Work out the finished part from the listing and answer in its coordinate system (mm). Face numbers are marked on the shaded views. A direction names the side the tool comes from. Give positions to 0.01 mm unless a question says otherwise; leave off trailing zeros. Write each loop counter-clockwise with the first axis right and the second up, starting at its lowest first coordinate (ties: lowest second). Pieces come first, ordered by that corner, then holes. Notation, with made-up numbers: (19, 51) -> (23, 51) arc R10 ccw to (23, 70) -> close; hole circle Ø1 at (-7, -36). An arc over 180 degrees is marked (long way). Write item = value, one per line. Start each with the question number.
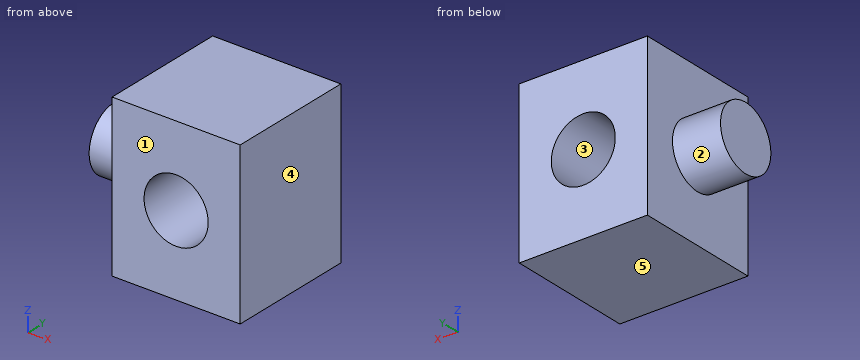
from build123d import *

# Parameters (mm, degrees)
F0_R     = 10
F1_DEPTH = 15
F0_W     = 40
F0_H     = 50
F2_DEPTH = 40
F3_R     = 10
F4_DEPTH = 40.001


with BuildPart() as f1:
    # F0 (on Right) → F1 (new body)
    with BuildSketch(Plane.YZ):
        Circle(F0_R)
    extrude(amount=-F1_DEPTH)

    # F0 (on Right) → F2 (join)
    with BuildSketch(Plane.YZ):
        Rectangle(F0_W, F0_H)
        Circle(F0_R, mode=Mode.SUBTRACT)
        Circle(F0_R)
    extrude(amount=F2_DEPTH)

    # F3 (on face) → F4 (cut, through all)
    with BuildSketch(Plane.XZ.offset(20)):
        with Locations((20, 0)):
            Circle(F3_R)
    extrude(amount=-F4_DEPTH, mode=Mode.SUBTRACT)


solid = f1.part
(1) Each of these flat-tipped pins is pushed along its axis until it touches: pin 1 (3 mm diameter, centred on x = -2.5, z = 16, fed in from -Y); pin 2 (1 mm diameter, centred on y = 15.5, z = 5.5, fed in from -X). Where does it stop, or does it pass through?
(2) Determine the mould class of the marked faces 3, 4 and 5 for opening direction Z: pulls with the +Z half, pulls with the -Z half, needs draft (parallel to the pull), parting line crosses it, or undercut.
(3) A cutting plane is placed at D-D, the plane y = -7.5. Write down the section's boundary in (x, z), then the cut area to 3 significant figures.
(4) Find the intervals of material crossed by line 1 along Z through (x, y) = (20, 2.5); line 2 along X through (y, z) = (-0.5, 13); line 3 along X through (y, z) = (8.5, -3.5), in increasing order.
(5) For the marked faces 1 and 2, determine the directions among +Z, -Z, +X, -X, +Y, -Y from which every point of the face is accessible in a straight line to the end or side of a thin tool.
(6) A cutting plane is placed at B-B, the plane x = 20. Write down the section's boundary in (y, z), then the cut area to 3 significant figures.
(7) A cutting plane is placed at A-A, the plane z = 0. Write down the section's boundary in (x, y).
(8) A cutting plane is placed at C-C, the plane y = 0. Write down the section's boundary in (x, z), then the cut area to 3 significant figures.
Results list:
q1.pin_1 = through
q1.pin_2 = 0
q2.face_3 = undercut
q2.face_4 = needs draft
q2.face_5 = pulls with the -Z half
q3.outline = (-15, -6.61) -> (0, -6.61) -> (0, -25) -> (40, -25) -> (40, 25) -> (0, 25) -> (0, 6.61) -> (-15, 6.61) -> close; hole circle Ø20 at (20, 0)
q3.area = 1,880 mm²
q4.line_1 = -25 to -10, 10 to 25
q4.line_2 = 0 to 40
q4.line_3 = -15 to 10.63, 29.37 to 40
q5.face_1 = +Z, -Z, +X, -X, -Y
q5.face_2 = -X
q6.outline = (-20, -25) -> (20, -25) -> (20, -10) -> (-20, -10) -> close; (-20, 10) -> (20, 10) -> (20, 25) -> (-20, 25) -> close
q6.area = 1,200 mm²
q7.outline = (-15, -10) -> (0, -10) -> (0, -20) -> (10, -20) -> (10, 20) -> (0, 20) -> (0, 10) -> (-15, 10) -> close; (30, -20) -> (40, -20) -> (40, 20) -> (30, 20) -> close
q8.outline = (-15, -10) -> (0, -10) -> (0, -25) -> (40, -25) -> (40, 25) -> (0, 25) -> (0, 10) -> (-15, 10) -> close; hole circle Ø20 at (20, 0)
q8.area = 1,990 mm²
